```python
from build123d import *

# Parameters (mm, degrees)
SKETCH1_R           = 1
BOSS_EXTRUDE1_DEPTH = 12.5
SKETCH2_R           = 2.25
BOSS_EXTRUDE2_DEPTH = 1
SKETCH3_W           = 0.6
SKETCH3_H           = 8.393754192
CUT_EXTRUDE1_DEPTH  = 0.35
FILLET1_R           = 0.05
FILLET2_R           = 0.05
CHAMFER1_SIZE       = 0.05


with BuildPart() as part:
    # Sketch1 → Boss-Extrude1 (new body)
    with BuildSketch(Plane.XY):
        Circle(SKETCH1_R)
    extrude(amount=BOSS_EXTRUDE1_DEPTH)

    # Sketch2 → Boss-Extrude2 (add)
    with BuildSketch(Plane.XY):
        Circle(SKETCH2_R)
    extrude(amount=-BOSS_EXTRUDE2_DEPTH)

    # Sketch3 → Cut-Extrude1 (cut)
    with BuildSketch(Plane(origin=(0, 0, -1), x_dir=(-1, 0, 0), z_dir=(0, 0, -1))):
        Rectangle(SKETCH3_W, SKETCH3_H)
    extrude(amount=-CUT_EXTRUDE1_DEPTH, mode=Mode.SUBTRACT)

    # Fillet1
    fillet1_edges = [part.edges().sort_by_distance(p)[0] for p in [
        (-2.25, 0, -1),
        (1.693738469, -1.481131324, -1),
        (0.3, 0, -1),
        (-0.3, 0, -1),
        (0, 2.25, -0.65),
        (0, -2.25, -0.65),
        (-0.3, -2.229910312, -0.825),
        (-0.3, 2.229910312, -0.825),
        (0.3, 2.229910312, -0.825),
        (0.3, -2.229910312, -0.825),
        (-0.3, 0, -0.65),
        (0.3, 0, -0.65),
        (-1, 0, 0),
    ]]
    fillet(fillet1_edges, radius=FILLET1_R)

    # Fillet2
    fillet2_edges = [part.edges().sort_by_distance(p)[0] for p in [
        (-2.25, 0, 0),
    ]]
    fillet(fillet2_edges, radius=FILLET2_R)

    # Chamfer1
    chamfer1_edges = [part.edges().sort_by_distance(p)[0] for p in [
        (-1, 0, 12.5),
    ]]
    chamfer(chamfer1_edges, length=CHAMFER1_SIZE)


solid = part.part
```
Geometry check sheet. Reference: the model listing, model coordinates, mm. A direction names the side the tool comes from. Coordinates: 2 decimals unless noted, no trailing zeros. Order: outer loops, then holes, each group sorted by start corner. A loop starts at its lowest first (then second) coordinate and runs counter-clockwise, first axis right, second up. Notation, with made-up numbers: M -30.75,30.25 L 13.25,30.25 A27 cw 13.25,56.25 Z; hole C 85,60.25 d3. An arc over 180 degrees is marked long. One line per question, with ' | ' between items. Start each with the question number.
Item 1: Set-up check for faces 1 (the flat face through (-1, 0, -1)), 2 (the cylindrical face through (0, -1, 6)): record each of +Z, -Z, +X, -X, +Y, -Y from which the full face is reachable in a straight line by a thin tool's end or side.
Item 2: Cross-section at B-B on y = 0. Enter the section's corners in (x, z).
Item 3: Cross-section at C-C on z = 0.5. Enter the section's corners in (x, y), then the cut area to 3 significant figures.
Item 4: Cross-section at A-A on x = 0. Enter the section's corners in (y, z), then the cut area to 3 significant figures.
Item 5: Gauge pin test, flat ends, axial feed: pin 1 (2 mm diameter, centred on y = -1, z = 8, fed in from -X); pin 2 (1.5 mm diameter, centred on x = -0.5, z = 9.5, fed in from +Y); pin 3 (1.5 mm diameter, centred on x = 0.5, z = 2, fed in from -Y); pin 4 (2 mm diameter, centred on x = -1.5, y = 1, fed in from +Z). Record the tip position at first contact, or that the pin passes through.
Item 6: Material ranges on L1, parallel to Z at x = -1.8, y = -1.2; L2, parallel to Z at x = 0.05, y = -1.6; L3, parallel to Y at x = -0.65, z = 1, recorded low to high. Write a range as [from, to].
Findings:
1) face 1: -Z, +X, -X, +Y, -Y | face 2: +Z
2) outline: M -2.25,-0.95 A0.05 ccw -2.2,-1 L -0.35,-1 A0.05 ccw -0.3,-0.95 L -0.3,-0.7 A0.05 cw -0.25,-0.65 L 0.25,-0.65 A0.05 cw 0.3,-0.7 L 0.3,-0.95 A0.05 ccw 0.35,-1 L 2.2,-1 A0.05 ccw 2.25,-0.95 L 2.25,-0.05 A0.05 ccw 2.2,0 L 1.05,0 A0.05 cw 1,0.05 L 1,12.45 L 0.95,12.5 L -0.95,12.5 L -1,12.45 L -1,0.05 A0.05 cw -1.05,0 L -2.2,0 A0.05 ccw -2.25,-0.05 Z
3) outline: C 0,0 d2 | area: 3.14 mm²
4) outline: M -2.25,-0.6 A0.05 ccw -2.2,-0.65 L 2.2,-0.65 A0.05 ccw 2.25,-0.6 L 2.25,-0.05 A0.05 ccw 2.2,0 L 1.05,0 A0.05 cw 1,0.05 L 1,12.45 L 0.95,12.5 L -0.95,12.5 L -1,12.45 L -1,0.05 A0.05 cw -1.05,0 L -2.2,0 A0.05 ccw -2.25,-0.05 Z | area: 27.9 mm²
5) pin 1: stops at x = -1 | pin 2: stops at y = 1 | pin 3: stops at y = -1 | pin 4: stops at z = 12.5
6) L1: z = [-1, 0] | L2: z = [-0.65, 0] | L3: y = [-0.76, 0.76]
